The listing builds one solid part. Answer for the finished solid, in the listing's coordinates (mm). A direction names the side the tool comes from. Round coordinates to 2 decimals unless told otherwise and drop trailing zeros. Loops run counter-clockwise (first coordinate to the right, second up) from the corner with the lowest first, then second, coordinate; pieces in that order, holes last. Notation, with made-up numbers: M 52,34.5 L 74,34.5 A21 ccw 74,38.5 Z; hole C 20.25,78.5 d2. An arc over 180 degrees is marked long. Answer as a JSON object with one key per item and string values.
```python
from build123d import *

# Parameters (mm, degrees)
ESQUISSE1_W             = 111.6
ESQUISSE1_H             = 25.9
BOSS_EXTRU_1_DEPTH      = 2
ESQUISSE2_W             = 7
ESQUISSE2_H             = 7
BOSS_EXTRU_2_DEPTH      = 16
ENL_V_MAT_EXTRU_1_DEPTH = 2


with BuildPart() as part:
    # Esquisse1 → Boss.-Extru.1 (new body)
    with BuildSketch(Plane.XY):
        with Locations((55.8, 12.95)):
            Rectangle(ESQUISSE1_W, ESQUISSE1_H)
    extrude(amount=BOSS_EXTRU_1_DEPTH)

    # Esquisse2 → Boss.-Extru.2 (add)
    with BuildSketch(Plane.XY.offset(2)):
        with Locations((41.5, 12.95)):
            Rectangle(ESQUISSE2_W, ESQUISSE2_H)
    extrude(amount=BOSS_EXTRU_2_DEPTH)

    # Esquisse3 → Enlèv. mat.-Extru.1 (cut)
    with BuildSketch(Plane(origin=(0, 0, 0), x_dir=(-1, 0, 0), z_dir=(0, 0, -1))):
        with BuildLine():
            Line((-111.6, 7.95), (-111.6, 17.95))
            ThreePointArc((-111.6, 17.95), (-109.528932188, 12.95), (-111.6, 7.95))
        make_face()
    extrude(amount=-ENL_V_MAT_EXTRU_1_DEPTH, mode=Mode.SUBTRACT)


solid = part.part
```
Item 1: Flat-ended cylindrical pins translate along their axes: P1, Ø13, axis at x = 81.5, y = 19.5, coming from the +Z side; P2, Ø3.5, axis at x = 40, z = 12, coming from the -Y side; P3, Ø5.5, axis at y = 11.5, z = 12.5, coming from the +X side. Find the tip coordinate at first contact, or state that the pin passes through.
Values follow:
{"P1": "z = 2", "P2": "y = 9.45", "P3": "x = 45"}
Item 2: Straight lines are drawn through the part: line 1 (Z direction, x = 10, y = 20); line 2 (X direction, y = 10.25, z = 8.75); line 3 (Y direction, x = 38.5, z = 11.75). For each, find the intervals that lie inside material, in ascending order.
Values follow:
{"line 1": "0 to 2", "line 2": "38 to 45", "line 3": "9.45 to 16.45"}
Item 3: The part is cut by section A-A (y = 11.25). Give the vertices of the cut face in (x, z).
Values follow:
{"outline": "M 0,0 L 109.74,0 L 109.74,2 L 45,2 L 45,18 L 38,18 L 38,2 L 0,2 Z"}
Item 4: The part is cut by section B-B (z = 16). Give the vertices of the cut face in (x, y), then the cut area to 3 significant figures.
Values follow:
{"outline": "M 38,9.45 L 45,9.45 L 45,16.45 L 38,16.45 Z", "area": "49.0 mm^2"}
Item 5: The part is cut by section C-C (x = 82). Give the vertices of the cut face in (y, z).
Values follow:
{"outline": "M 0,0 L 25.9,0 L 25.9,2 L 0,2 Z"}
Item 6: Which of the six approach directions +Z, -Z, +X, -X, +Y, -Y give full straight-line access (tool end or side, diameter ignored) to faces 1 (the face through (41, 9.45, 10)), 2 (the face through (45, 13, 10)), 3 (the face through (38, 13, 10)), 4 (the face through (41, 16.45, 10))?
Values follow:
{"face 1": "+Z, +X, -X, -Y", "face 2": "+Z, +X, +Y, -Y", "face 3": "+Z, -X, +Y, -Y", "face 4": "+Z, +X, -X, +Y"}
